```python
from build123d import *

# Parameters (mm, degrees)
PAD004_DEPTH    = 30
PAD005_DEPTH    = 20
SKETCH019_R     = 2.1
POCKET007_DEPTH = 55.4884980464
SKETCH020_R     = 2.6
POCKET008_DEPTH = 39.001
SKETCH021_R     = 4.75
POCKET009_DEPTH = 9.5
PAD007_DEPTH    = 38
SKETCH026_R     = 1.5
POCKET012_DEPTH = 4


with BuildPart() as part:
    # Sketch017 (on DatumPlane) → Pad004 (new body)
    with BuildSketch(Plane(origin=(0, 0, -127.29162), x_dir=(1, 0, 0), z_dir=(0, 0, -1))):
        with BuildLine():
            ThreePointArc((-1, 6.9282032303), (-7, 0), (-1, -6.9282032303))
            Line((-1, -6.9282032303), (-1, -39.9874980463))
            ThreePointArc((-1, 39.9874980463), (-40, 0), (-1, -39.9874980463))
            Line((-1, 6.9282032303), (-1, 39.9874980463))
        make_face()
    extrude(amount=PAD004_DEPTH)

    # Sketch018 (on Face5 of Pad004) → Pad005 (join)
    with BuildSketch(Plane.XY.offset(-127.29162)):
        with BuildLine():
            ThreePointArc((-29.5109069739, -5.5), (-28.0584714971, -10.6707922701), (-25.7078515326, -15.5))
            Line((-25.7078515327, -15.5), (-13.7078515327, -15.5))
            Line((-13.7078515327, -15.5), (-13.7078515327, -5.5))
            Line((-13.7078515327, -5.5), (-29.5109069739, -5.5))
        make_face()
    pad005 = extrude(amount=PAD005_DEPTH)

    # Mirrored: Pad005 across Sketch018 H_Axis
    add(pad005.mirror(Plane(origin=(0, 0, -127.29162), x_dir=(0, 0, 1), z_dir=(0, 1, 0))))

    # Sketch019 (on Face10 of Mirrored) → Pocket007 (cut, through all)
    with BuildSketch(Plane(origin=(0, -15.5, -127.29162), x_dir=(-1, 0, 0), z_dir=(0, -1, 0))):
        with Locations((19.005882937, -11)):
            Circle(SKETCH019_R)
    extrude(amount=-POCKET007_DEPTH, mode=Mode.SUBTRACT)

    # Sketch020 (on Face2 of Pocket007) → Pocket008 (cut, through all)
    with BuildSketch(Plane(origin=(-1, 0, -127.29162), x_dir=(0, -1, 0), z_dir=(1, 0, 0))):
        with Locations((-23.4578506383, 15)):
            Circle(SKETCH020_R)
        with Locations((23.4578506383, 15)):
            Circle(SKETCH020_R)
    extrude(amount=-POCKET008_DEPTH, mode=Mode.SUBTRACT)

    # Sketch021 (on DatumPlane) → Pocket009 (cut, symmetric)
    with BuildSketch(Plane(origin=(-33, -23.4578506383, -142.29162), x_dir=(0, 0, 1), z_dir=(1, 0, 0))):
        with Locations((0, -46.9157012765)):
            Circle(SKETCH021_R)
        Circle(SKETCH021_R)
    extrude(amount=POCKET009_DEPTH, both=True, mode=Mode.SUBTRACT)

    # Sketch025 (on DatumPlane) → Pad007 (join)
    with BuildSketch(Plane(origin=(0, 0, -127.29162), x_dir=(1, 0, 0), z_dir=(0, 0, -1))):
        with BuildLine():
            Line((-12.8257553747, 35.2384732795), (-11.4576748014, 31.4797027963))
            ThreePointArc((-11.4576748014, 31.4797027963), (-15.4685785433, 29.7148629115), (-19.2148106176, 27.4415934838))
            Line((-21.509116363, 30.7182016609), (-19.2148106176, 27.4415934838))
            ThreePointArc((-12.8257553747, 35.2384732795), (-17.3155729962, 33.2629062442), (-21.509116363, 30.7182016609))
        make_face()
    extrude(amount=-PAD007_DEPTH)

    # Sketch026 (on DatumPlane) → Pocket012 (cut, symmetric)
    with BuildSketch(Plane(origin=(-17.2661657333, -33.1679957752, -108.29162), x_dir=(0.8870108332, -0.4617486132, 0), z_dir=(0.4617486132, 0.8870108332, 0))):
        with Locations((0, -16.226432)):
            Circle(SKETCH026_R)
    extrude(amount=POCKET012_DEPTH, both=True, mode=Mode.SUBTRACT)


solid = part.part
```
Input: part model. Units: mm. Frame: model coordinates. A direction names the side the tool comes from. Coordinates: 2 decimals unless noted, no trailing zeros. Write each loop counter-clockwise with the first axis right and the second up, starting at its lowest first coordinate (ties: lowest second). Pieces come first, ordered by that corner, then holes. Notation, with made-up numbers: (12, 61) -> (31, 61) arc R27 cw to (31, 81) -> close; hole circle Ø8 at (-2, 27). An arc over 180 degrees is marked (long way). Write each question's results on one line, items separated by ' | '.
Item 1: Section query D-D on y = 0. Return loops of the section in (x, z).
Conclusion:
outline: (-40, -157.29) -> (-7, -157.29) -> (-7, -127.29) -> (-40, -127.29) -> close
Item 2: Pin query (flat end, axial travel): pin 1 Ø5 at (x, y) = (-21.5, 9) entering from +Z; pin 2 Ø5 at (x, z) = (-10, -146.5) entering from +Y; pin 3 Ø12.5 at (x, z) = (-18, -112.5) entering from +Y. Return the tip coordinate at first contact, or that it passes through.
Conclusion:
pin 1: stops at z = -107.29 | pin 2: stops at y = 39.29 | pin 3: stops at y = 15.5
Item 3: Section query A-A on y = -14.5. Return loops of the section in (x, z).
Conclusion:
outline: (-37.28, -157.29) -> (-1, -157.29) -> (-1, -127.29) -> (-13.71, -127.29) -> (-13.71, -107.29) -> (-26.28, -107.29) -> (-26.28, -127.29) -> (-37.28, -127.29) -> close; hole circle Ø4.2 at (-19.01, -116.29)
Item 4: Set-up query: faces 1 (the cylindrical face through (-15.414, -29.743, -108.558)), 2 (the cylindrical face through (-17.255, -33.295, -108.558)), 3 (the flat face through (-23.5, -21, -140)), 4 (the flat face through (-21.1, 15.5, -117.4)). Return all of +Z, -Z, +X, -X, +Y, -Y with unobstructed straight access to the full face (end or side cutting, diameter ignored); none if empty.
Conclusion:
face 1: +Z, +X | face 2: +Z, -X, -Y | face 3: -X | face 4: +Z, +X, -X, +Y
Item 5: Section query B-B on x = -34. Return loops of the section in (y, z), plus the area to 3 significant figures.
Conclusion:
outline: (-21.07, -157.29) -> (21.07, -157.29) -> (21.07, -146.4) arc R4.75 cw to (21.07, -138.18) -> (21.07, -127.29) -> (-21.07, -127.29) -> (-21.07, -138.18) arc R4.75 cw to (-21.07, -146.4) -> close | area: 1,240 mm^2
Item 6: Material intervals for probe 1 along Y at (x, z) = (-16, -108); probe 2 along Y at (x, z) = (-21, -124.5); probe 3 along Z at (x, y) = (-11.5, -29), sorted ascending.
Conclusion:
probe 1: y = -33.92 to -29.43, -15.5 to -5.5, 5.5 to 15.5 | probe 2: y = -31.07 to -29.99, -15.5 to -5.5, 5.5 to 15.5 | probe 3: z = -157.29 to -127.29
Item 7: Section query C-C on z = -130.5. Return loops of the section in (x, y), plus the area to 3 significant figures.
Conclusion:
outline: (-1, -39.99) -> (-1, -6.93) arc R7 cw to (-1, 6.93) -> (-1, 39.99) arc R40 ccw to start | area: 2,370 mm^2
Item 8: Mould query, pull axis Z, two halves, no side actions, for faces 5 (the flat face through (-16, -1, -157.292)), 6 (the flat face through (-1, -23.2, -145.4)), 7 (the cylindrical face through (-20.135, 10.43, -118.062)). Classes: +Z half, -Z half, draft (parallel to the pull), parting line (faces both ways), or undercut.
Conclusion:
face 5: -Z half | face 6: draft | face 7: undercut
